The listing builds one solid part. Answer for the finished solid, in the listing's coordinates (mm). A direction names the side the tool comes from. Round coordinates to 2 decimals unless told otherwise and drop trailing zeros. Loops run counter-clockwise (first coordinate to the right, second up) from the corner with the lowest first, then second, coordinate; pieces in that order, holes last. Notation, with made-up numbers: (4.25, 30.25) -> (30.25, 30.25) arc R23 cw to (30.25, 65.25) -> close; hole circle Ø10 at (-1, 62.5). An arc over 180 degrees is marked (long way). Use a Markdown table: item, result. Add a question column.
Q1. Section A-A on x = 50 is taken. Give the vertices of the cut face in (y, z).
Q2. Section B-B on z = -26.67 is taken. Give the vertices of the cut face in (x, y), then the cut area to 3 significant figures.
Q3. Consider line 1 (Y direction, x = 26, z = -18.5); line 2 (Z direction, x = 50.8, y = -3.25); line 3 (Z direction, x = 9, y = -27.5). Determine where each line is inside the solid, lowest interval first.
Q4. Section D-D on x = 85.5 is taken. Give the vertices of the cut face in (y, z).
Q5. Which of the six approach directions +Z, -Z, +X, -X, +Y, -Y give full straight-line access (tool end or side, diameter ignored) to faces 5 (the flat face through (52, -6.35, -17)), 6 (the flat face through (0, -24, -6))?
Q6. Section C-C on z = -10.5 is taken. Give the vertices of the cut face in (x, y), then the cut area to 3 significant figures.
Q7. For a pull along Z with two mould halves and no side action, classify faces 1 (the flat face through (52, -38.1, -17)), 2 (the flat face through (50, -22, 0)), 3 (the flat face through (50, -41, -44.45)), 4 (the cylindrical face through (56.666, -41.319, -29.102)) as released by +Z, released by -Z, zero draft, split by the parting line, or undercut.
Q8. Given pin 1 Ø16 at (x, y) = (44, -22.5) entering from -Z, flat-ended and moving along its own axis, determine where the tip first touches the part or whether it passes through.
from build123d import *

# Parameters (mm, degrees)
F0_W     = 101.6
F0_H     = 44.45
F1_DEPTH = 44.45
F2_W     = 31.75
F2_H     = 38.1
F3_DEPTH = 101.601
F4_R     = 6.35
F5_DEPTH = 44.451


with BuildPart() as f1:
    # F0 (on Front) → F1 (new body)
    with BuildSketch(Plane.XZ):
        with Locations((50.8, -22.225)):
            Rectangle(F0_W, F0_H)
    extrude(amount=F1_DEPTH)

    # F2 (on face) → F3 (cut, through all)
    with BuildSketch(Plane.YZ.offset(101.6)):
        with Locations((-22.225, -25.4)):
            Rectangle(F2_W, F2_H)
    extrude(amount=-F3_DEPTH, mode=Mode.SUBTRACT)

    # F4 (on face) → F5 (cut, through all)
    with BuildSketch(Plane.XZ.offset(44.45)):
        with Locations((50.8, -26.67)):
            Circle(F4_R)
    extrude(amount=-F5_DEPTH, mode=Mode.SUBTRACT)


solid = f1.part
Checked values:
| question | item | result |
|---|---|---|
| 1 | outline | (-44.45, -44.45) -> (-38.1, -44.45) -> (-38.1, -32.97) -> (-44.45, -32.97) -> close; (-44.45, -20.37) -> (-38.1, -20.37) -> (-38.1, -6.35) -> (-6.35, -6.35) -> (-6.35, -20.37) -> (0, -20.37) -> (0, 0) -> (-44.45, 0) -> close; (-6.35, -44.45) -> (0, -44.45) -> (0, -32.97) -> (-6.35, -32.97) -> close |
| 2 | outline | (0, -44.45) -> (44.45, -44.45) -> (44.45, -38.1) -> (0, -38.1) -> close; (0, -6.35) -> (44.45, -6.35) -> (44.45, 0) -> (0, 0) -> close; (57.15, -44.45) -> (101.6, -44.45) -> (101.6, -38.1) -> (57.15, -38.1) -> close; (57.15, -6.35) -> (101.6, -6.35) -> (101.6, 0) -> (57.15, 0) -> close |
| 2 | area | 1,130 mm2 |
| 3 | line 1 | y = -44.45 to -38.1, -6.35 to 0 |
| 3 | line 2 | z = -44.45 to -33.02, -20.32 to 0 |
| 3 | line 3 | z = -6.35 to 0 |
| 4 | outline | (-44.45, -44.45) -> (-38.1, -44.45) -> (-38.1, -6.35) -> (-6.35, -6.35) -> (-6.35, -44.45) -> (0, -44.45) -> (0, 0) -> (-44.45, 0) -> close |
| 5 | face 5 | -Z, +X, -X |
| 5 | face 6 | +Z, -Z, -X, +Y, -Y |
| 6 | outline | (0, -44.45) -> (101.6, -44.45) -> (101.6, -38.1) -> (0, -38.1) -> close; (0, -6.35) -> (101.6, -6.35) -> (101.6, 0) -> (0, 0) -> close |
| 6 | area | 1,290 mm2 |
| 7 | face 1 | zero draft |
| 7 | face 2 | released by +Z |
| 7 | face 3 | released by -Z |
| 7 | face 4 | undercut |
| 8 | pin 1 | stops at z = -6.35 |
